Geometry: final body of the model. Coordinates: model frame, mm. A direction names the side the tool comes from. Give positions to 0.01 mm unless a question says otherwise; leave off trailing zeros. Write each loop counter-clockwise with the first axis right and the second up, starting at its lowest first coordinate (ties: lowest second). Pieces come first, ordered by that corner, then holes. Notation, with made-up numbers: M 80.5,81.5 L 128.5,81.5 A19 cw 128.5,114.5 Z; hole C 79.25,-38 d10. An arc over 180 degrees is marked long. Answer as a JSON object with one key per item and string values.
Autodesk Inventor part; units mm, degrees
ref_plane "conn_XY" through (0, 0, 0) normal (0, 0, -1) x (1, 0, 0)
ref_plane "conn_YZ" through (0, 0, 0) normal (1, 0, 0) x (0, -1, 0)
ref_plane "conn_ZX" through (0, 0, 0) normal (0, -1, 0) x (0, 0, -1)
sketch "Sketch_1" plane through (0, 0, 0) normal (1, 0, 0) x (0, 1, 0)
  line L0 (0, -208.1721) -> (0, 12.7)
  line L1 (0, 12.7) -> (2.634, 12.7)
  line L2 (2.634, 12.7) -> (3.175, 12.159)
  line L3 (3.175, 12.159) -> (3.175, 0)
  line L4 (3.175, 0) -> (4.0005, -0.8255)
  line L5 (4.0005, -0.8255) -> (4.0005, -198.6471)
  line L6 (4.0005, -198.6471) -> (9.5123, -198.6471)
  line L7 (9.5123, -198.6471) -> (9.5123, -208.1721)
  line L8 (9.5123, -208.1721) -> (0, -208.1721)
  line L9 (0, -208.1721) -> (0, 12.7)
revolve "Revolution1" add sketch "Sketch_1" angle 360 about axis through (0, 0, -208.1721) along (0, 0, -1)
thread "Thread1"
sketch "Sketch_2" plane through (0, 0, 0) normal (1, 0, 0) x (0, 1, 0)
  line L0 (6.096, 0) -> (3.048, 0)
  line L1 (3.048, 0) -> (3.048, -3.9878)
  line L2 (3.048, -3.9878) -> (6.096, -7.0358)
  line L3 (6.096, -7.0358) -> (6.096, 0)
extrude "Extrusion1" cut sketch "Sketch_2" along normal mid plane 16.002
sketch "Sketch_3" plane through (0, 0, 0) normal (1, 0, 0) x (0, 1, 0)
  line L0 (-6.096, 0) -> (-6.096, -7.0358)
  line L1 (-6.096, -7.0358) -> (-3.048, -3.9878)
  line L2 (-3.048, -3.9878) -> (-3.048, 0)
  line L3 (-3.048, 0) -> (-6.096, 0)
extrude "Extrusion2" cut sketch "Sketch_3" along normal mid plane 16.002
ref_plane "conn_XY" through (0, 0, 0) normal (0, 0, -1) x (1, 0, 0)
ref_plane "conn_YZ" through (0, 0, 0) normal (1, 0, 0) x (0, -1, 0)
ref_plane "conn_ZX" through (0, 0, 0) normal (0, -1, 0) x (0, 0, -1)
properties part number "PR_OCG1-3/4x6" material "Stainless Steel"
1) Set-up query: faces 1 (the flat face through (0, 0, 12.7)), 2 (the cylindrical face through (-9.286, -2.062, -203.476)), 3 (the cylindrical face through (-3.9, -0.9, -101.1)). Return all of +Z, -Z, +X, -X, +Y, -Y with unobstructed straight access to the full face (end or side cutting, diameter ignored); none if empty.
Geometry check:
{"face 1": "+Z, +X, -X, +Y, -Y", "face 2": "+Z, -Z", "face 3": "+Z"}
2) Contact query for flat-ended pins moving along their axis: P1, Ø1.5, axis at x = 1.5, y = -3.5, coming from the +Z side; P2, Ø5, axis at y = -6, z = -140.5, coming from the -X side; P3, Ø4.5, axis at x = -1, z = -2.5, coming from the -Y side; P4, Ø1, axis at y = -5, z = -98, coming from the -X side. Output: stop coordinate, or through.
Geometry check:
{"P1": "stops at z = 12.28", "P2": "stops at x = -1.94", "P3": "stops at y = -3.81", "P4": "passes through"}
3) Cut plane A-A on y = 0. Return loops of the section in (x, z) (1 decimal), and give its area (3 significant figures).
Geometry check:
{"outline": "M -9.5,-208.2 L 9.5,-208.2 L 9.5,-198.6 L 4,-198.6 L 4,-0.8 L 3.2,0 L 3.2,12.2 L 2.6,12.7 L -2.6,12.7 L -3.2,12.2 L -3.2,0 L -4,-0.8 L -4,-198.6 L -9.5,-198.6 Z", "area": "1,850 mm2"}
4) Line query: line 1 (Y direction, x = -3, z = -183); line 2 (Z direction, x = -3.75, y = -4); line 3 (X direction, y = 0.25, z = -58.5). Output: solid intervals per line, ascending. Write a range as from..to.
Geometry check:
{"line 1": "y = -2.65..2.65", "line 2": "z = -208.17..-198.65", "line 3": "x = -3.99..3.99"}
5) Cut plane B-B on z = -25.5. Return loops of the section in (x, y).
Geometry check:
{"outline": "C 0,0 d8"}
